```python
from build123d import *

# Parameters (mm, degrees)
SKETCH1_W           = 40
SKETCH1_H           = 210
BOSS_EXTRUDE1_DEPTH = 25
SKETCH2_W           = 40
SKETCH2_H           = 25
BOSS_EXTRUDE2_DEPTH = 30
SKETCH3_W           = 40
SKETCH3_H           = 25
BOSS_EXTRUDE3_DEPTH = 30
BOSS_EXTRUDE4_DEPTH = 80
SKETCH6_W           = 20
SKETCH6_H           = 20
BOSS_EXTRUDE5_DEPTH = 120
SKETCH7_W           = 20
SKETCH7_H           = 20
BOSS_EXTRUDE6_DEPTH = 120
SKETCH8_W           = 20
SKETCH8_H           = 20
BOSS_EXTRUDE7_DEPTH = 70


with BuildPart() as part:
    # Sketch1 → Boss-Extrude1 (new body)
    with BuildSketch(Plane.XY):
        with Locations((20, 105)):
            Rectangle(SKETCH1_W, SKETCH1_H)
    extrude(amount=BOSS_EXTRUDE1_DEPTH)

    # Sketch2 → Boss-Extrude2 (add)
    with BuildSketch(Plane(origin=(0, 210, 0), x_dir=(1, 0, 0), z_dir=(0, 1, 0))):
        Polygon((0, 0), (-17.5, 0), (-17.5, -40), (57.5, -40), (57.5, 0), (40, 0), (40, -25), (0, -25), align=None)
        with Locations((20, -12.5)):
            Rectangle(SKETCH2_W, SKETCH2_H)
    extrude(amount=BOSS_EXTRUDE2_DEPTH)

    # Sketch3 → Boss-Extrude3 (add)
    with BuildSketch(Plane.XZ):
        Polygon((57.5, 40), (57.5, 0), (40, 0), (40, 25), (0, 25), (0, 0), (-17.5, 0), (-17.5, 40), align=None)
        with Locations((20, 12.5)):
            Rectangle(SKETCH3_W, SKETCH3_H)
    extrude(amount=BOSS_EXTRUDE3_DEPTH)

    # Sketch5 → Boss-Extrude4 (add)
    with BuildSketch(Plane(origin=(0, 50, 0), x_dir=(1, 0, 0), z_dir=(0, 1, 0))):
        Polygon((57.5, 0), (0, 0), (-17.5, 0), (-17.5, -40), (57.5, -40), align=None)
    extrude(amount=BOSS_EXTRUDE4_DEPTH)

    # Sketch6 → Boss-Extrude5 (add)
    with BuildSketch(Plane(origin=(11.25, 0, 11.25), x_dir=(0.707106781, 0, -0.707106781), z_dir=(0.707106781, 0, 0.707106781))):
        with Locations((-8.158639918, 100)):
            Rectangle(SKETCH6_W, SKETCH6_H)
    extrude(amount=BOSS_EXTRUDE5_DEPTH)

    # Sketch7 → Boss-Extrude6 (add)
    with BuildSketch(Plane(origin=(8.75, 0, -8.75), x_dir=(0.707106781, 0, 0.707106781), z_dir=(-0.707106781, 0, 0.707106781))):
        with Locations((36.442911166, 100)):
            Rectangle(SKETCH7_W, SKETCH7_H)
    extrude(amount=BOSS_EXTRUDE6_DEPTH)

    # Sketch8 → Boss-Extrude7 (add)
    with BuildSketch(Plane.XY.offset(94.800775542)):
        with Locations((-47.404851943, 100)):
            Rectangle(SKETCH8_W, SKETCH8_H)
        with Locations((87.404851943, 100)):
            Rectangle(SKETCH8_W, SKETCH8_H)
    extrude(amount=BOSS_EXTRUDE7_DEPTH)


solid = part.part
```
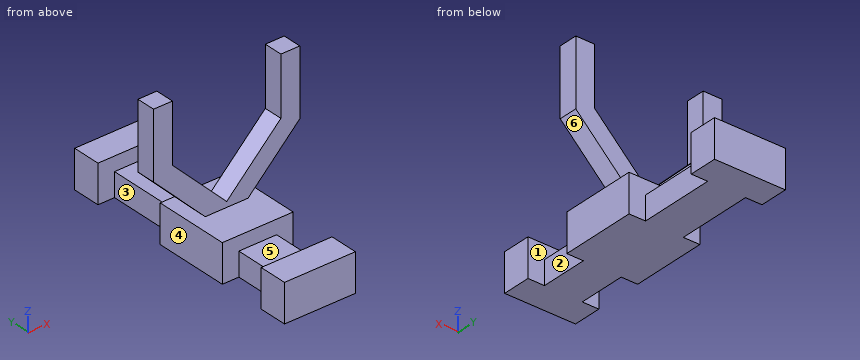
Design review of the part built by this model. Coordinates are the model's own, in mm. Face numbers are marked on the shaded views. A direction names the side the tool comes from. Round coordinates to 2 decimals unless told otherwise and drop trailing zeros. Order: outer loops, then holes, each group sorted by start corner. A loop starts at its lowest first (then second) coordinate and runs counter-clockwise, first axis right, second up. Notation, with made-up numbers: M 58,67 L 106,67 A9 cw 106,83 Z; hole C 25,74.25 d1. An arc over 180 degrees is marked long. Put each result on its own line as item: value.
Q1. Machinability: for the marked faces 1, 2 and 3, which of the approach directions +Z, -Z, +X, -X, +Y, -Y give a long, thin tool a straight path to every point of the face, cutting with its end or side? Answer none if there is none.
Reported:
face 1: +Z
face 2: +Z, -Z, +X
face 3: +Z, -Z, -X
Q2. Insertion check: pin 1 Ø12 at (x, y) = (31, 108.5) entering from -Z; pin 2 Ø9 at (y, z) = (231.5, 16) entering from +X; pin 3 Ø20 at (y, z) = (80.5, 29) entering from -X; pin 4 Ø4 at (x, y) = (16, 138.5) entering from +Z. Each pin has a flat end and moves straight along its axis. Give the tip position at first contact, or say it passes through.
Reported:
pin 1: z = 0
pin 2: x = 57.5
pin 3: x = -17.5
pin 4: z = 25
Q3. Consider section B-B (z = 128). State the section outline as (x, y) points, and give its area (3 significant figures).
Reported:
outline: M -57.4,90 L -37.4,90 L -37.4,110 L -57.4,110 Z; M 77.4,90 L 97.4,90 L 97.4,110 L 77.4,110 Z
area: 800 mm²
Q4. Draft analysis for pull direction Z (two halves, no side actions). For the marked faces 4, 5 and 6, state which applies: released by +Z, released by -Z, zero draft, split by the parting line, or undercut.
Reported:
face 4: zero draft
face 5: released by +Z
face 6: undercut
Q5. To check wall thickness, follow line 1 (Y direction, x = 15, z = 32.5); line 2 (X direction, y = 74, z = 11); line 3 (Z direction, x = -1.5, y = -10). State the ranges of each line that lie inside material, in increasing order.
Reported:
line 1: -30 to 0, 50 to 130, 210 to 240
line 2: -17.5 to 57.5
line 3: 0 to 40
Q6. Consider section D-D (z = 11.5). State the section outline as (x, y) points, and give its area (3 significant figures).
Reported:
outline: M -17.5,-30 L 57.5,-30 L 57.5,0 L 40,0 L 40,50 L 57.5,50 L 57.5,130 L 40,130 L 40,210 L 57.5,210 L 57.5,240 L -17.5,240 L -17.5,210 L 0,210 L 0,130 L -17.5,130 L -17.5,50 L 0,50 L 0,0 L -17.5,0 Z
area: 15,700 mm²
Q7. Consider section C-C (y = -4.5). State the section outline as (x, z) points.
Reported:
outline: M -17.5,0 L 57.5,0 L 57.5,40 L -17.5,40 Z
Q8. Consider section A-A (z = 31.5). State the section outline as (x, y) points.
Reported:
outline: M -17.5,-30 L 57.5,-30 L 57.5,0 L -17.5,0 Z; M -17.5,50 L 57.5,50 L 57.5,130 L -17.5,130 Z; M -17.5,210 L 57.5,210 L 57.5,240 L -17.5,240 Z
